from build123d import *

# Parameters (mm, degrees)
SKETCH_1_W          = 25
SKETCH_1_H          = 15
EXTRUDE_2_DEPTH     = 2
SKETCH_3_W          = 2
SKETCH_3_H          = 25
EXTRUDE_3_DEPTH     = 33
SKETCH_4_W          = 25
SKETCH_4_H          = 2
EXTRUDE_4_DEPTH     = 33
SKETCH_5_R          = 1
CUT_EXTRUDE_2_DEPTH = 71.75485849
SKETCH_6_R          = 1
CUT_EXTRUDE_3_DEPTH = 71.75485849
SKETCH_7_R          = 3
CUT_EXTRUDE_4_DEPTH = 71.75485849
SKETCH_8_R          = 3
CUT_EXTRUDE_5_DEPTH = 71.75485849
SKETCH_9_R          = 12.5
SKETCH_9_R_2        = 3
EXTRUDE_5_DEPTH     = 2
SKETCH_10_R         = 12.5
SKETCH_10_R_2       = 3
EXTRUDE_6_DEPTH     = 2
SKETCH_11_R         = 1
CUT_EXTRUDE_6_DEPTH = 71.75485849
SKETCH_12_R         = 12.5
SKETCH_12_R_2       = 3
EXTRUDE_7_DEPTH     = 2
EXTRUDE_START       = -2
SKETCH_13_R         = 12.5
SKETCH_13_R_2       = 3
EXTRUDE_8_DEPTH     = 2
SKETCH_14_R         = 1
CUT_EXTRUDE_7_DEPTH = 71.75485849


with BuildPart() as part:
    # 草图1 → 凸台-拉伸2 (new body)
    with BuildSketch(Plane.XY):
        Polygon((-12.5, 12.5), (-27.5, 12.5), (-27.5, -12.5), (-12.5, -12.5), (12.5, -12.5), (27.5, -12.5), (27.5, 12.5), (12.5, 12.5), align=None)
        with Locations((0, 20)):
            Rectangle(SKETCH_1_W, SKETCH_1_H)
        with Locations((0, -20)):
            Rectangle(SKETCH_1_W, SKETCH_1_H)
    extrude(amount=EXTRUDE_2_DEPTH)

    # 草图3 → 凸台-拉伸3 (add)
    with BuildSketch(Plane.XY.offset(2)):
        with Locations((26.5, 0)):
            Rectangle(SKETCH_3_W, SKETCH_3_H)
        with Locations((-26.5, 0)):
            Rectangle(SKETCH_3_W, SKETCH_3_H)
    extrude(amount=EXTRUDE_3_DEPTH)

    # 草图4 → 凸台-拉伸4 (add)
    with BuildSketch(Plane(origin=(0, 0, 0), x_dir=(-1, 0, 0), z_dir=(0, 0, -1))):
        with Locations((0, 26.5)):
            Rectangle(SKETCH_4_W, SKETCH_4_H)
        with Locations((0, -26.5)):
            Rectangle(SKETCH_4_W, SKETCH_4_H)
    extrude(amount=EXTRUDE_4_DEPTH)

    # 草图5 → 切除-拉伸2 (cut, through all)
    with BuildSketch(Plane.ZY.offset(27.5)):
        with BuildLine():
            Line((35, 12.5), (22.5, 12.5))
            ThreePointArc((22.5, 12.5), (31.338834765, 8.838834765), (35, 0))
            Line((35, 0), (35, 12.5))
        make_face()
        with BuildLine():
            Line((35, -12.5), (35, 0))
            ThreePointArc((35, 0), (31.338834765, -8.838834765), (22.5, -12.5))
            Line((22.5, -12.5), (35, -12.5))
        make_face()
        with Locations((29.682514636, 0)):
            Circle(SKETCH_5_R)
        with Locations((22.5, 6.957836122)):
            Circle(SKETCH_5_R)
        with Locations((15.317485364, 0)):
            Circle(SKETCH_5_R)
        with Locations((22.5, -6.957836122)):
            Circle(SKETCH_5_R)
    extrude(amount=-CUT_EXTRUDE_2_DEPTH, mode=Mode.SUBTRACT)

    # 草图6 → 切除-拉伸3 (cut, through all)
    with BuildSketch(Plane(origin=(0, 27.5, 0), x_dir=(1, 0, 0), z_dir=(0, 1, 0))):
        with BuildLine():
            Line((-12.5, 33), (-12.5, 20.5))
            ThreePointArc((-12.5, 20.5), (-8.838834765, 29.338834765), (0, 33))
            Line((0, 33), (-12.5, 33))
        make_face()
        with BuildLine():
            ThreePointArc((0, 33), (8.838834765, 29.338834765), (12.5, 20.5))
            Line((12.5, 20.5), (12.5, 33))
            Line((12.5, 33), (0, 33))
        make_face()
        with Locations(Location((6.473248516, 20.5, 0), (0, 0, 270))):
            Circle(SKETCH_6_R)
        with Locations(Location((0, 28.122142327, 0), (0, 0, 270))):
            Circle(SKETCH_6_R)
        with Locations(Location((-6.473248516, 20.5, 0), (0, 0, 270))):
            Circle(SKETCH_6_R)
        with Locations(Location((0, 12.877857673, 0), (0, 0, 270))):
            Circle(SKETCH_6_R)
    extrude(amount=-CUT_EXTRUDE_3_DEPTH, mode=Mode.SUBTRACT)

    # 草图7 → 切除-拉伸4 (cut, through all)
    with BuildSketch(Plane(origin=(0, 27.5, 0), x_dir=(1, 0, 0), z_dir=(0, 1, 0))):
        with Locations(Location((0, 20.5, 0), (0, 0, 270))):
            Circle(SKETCH_7_R)
    extrude(amount=-CUT_EXTRUDE_4_DEPTH, mode=Mode.SUBTRACT)

    # 草图8 → 切除-拉伸5 (cut, through all)
    with BuildSketch(Plane(origin=(27.5, 0, 0), x_dir=(0, 0, -1), z_dir=(1, 0, 0))):
        with Locations((-22.5, 0)):
            Circle(SKETCH_8_R)
    extrude(amount=-CUT_EXTRUDE_5_DEPTH, mode=Mode.SUBTRACT)

    # 草图9 → 凸台-拉伸5 (add)
    with BuildSketch(Plane(origin=(27.5, 0, 0), x_dir=(0, 0, -1), z_dir=(1, 0, 0))):
        with Locations((-22.5, 0)):
            Circle(SKETCH_9_R)
        with Locations((-22.5, 0)):
            Circle(SKETCH_9_R_2, mode=Mode.SUBTRACT)
    extrude(amount=-EXTRUDE_5_DEPTH)

    # 草图10 → 凸台-拉伸6 (add)
    with BuildSketch(Plane.ZY.offset(27.5)):
        with Locations((22.5, 0)):
            Circle(SKETCH_10_R)
        with Locations(Location((22.5, 0, 0), (0, 0, 180))):
            Circle(SKETCH_10_R_2, mode=Mode.SUBTRACT)
    extrude(amount=-EXTRUDE_6_DEPTH)

    # 草图11 → 切除-拉伸6 (cut, through all)
    with BuildSketch(Plane.ZY.offset(27.5)):
        with Locations((22.5, 7.071067812)):
            Circle(SKETCH_11_R)
        with Locations((29.571067812, 0)):
            Circle(SKETCH_11_R)
        with Locations(Location((22.5, -7.071067812, 0), (0, 0, 90))):
            Circle(SKETCH_11_R)
        with Locations(Location((15.428932188, 0, 0), (0, 0, 90))):
            Circle(SKETCH_11_R)
    extrude(amount=-CUT_EXTRUDE_6_DEPTH, mode=Mode.SUBTRACT)

    # 草图12 → 凸台-拉伸7 (add)
    with BuildSketch(Plane(origin=(0, 27.5, 0), x_dir=(1, 0, 0), z_dir=(0, 1, 0))):
        with Locations((0, 20.5)):
            Circle(SKETCH_12_R)
        with Locations(Location((0, 20.5, 0), (0, 0, 270))):
            Circle(SKETCH_12_R_2, mode=Mode.SUBTRACT)
    extrude(amount=-EXTRUDE_7_DEPTH)

    # 草图13 → 凸台-拉伸8 (add)
    with BuildSketch(Plane.XZ.offset(27.5).offset(EXTRUDE_START)):
        with Locations((0, -20.5)):
            Circle(SKETCH_13_R)
        with Locations(Location((0, -20.5, 0), (0, 0, 90))):
            Circle(SKETCH_13_R_2, mode=Mode.SUBTRACT)
    extrude(amount=EXTRUDE_8_DEPTH)

    # 草图14 → 切除-拉伸7 (cut, through all)
    with BuildSketch(Plane(origin=(0, -27.5, 0), x_dir=(-1, 0, 0), z_dir=(0, -1, 0))):
        with Locations(Location((0, 13.428932188, 0), (0, 0, 90))):
            Circle(SKETCH_14_R)
        with Locations(Location((-7.071067812, 20.5, 0), (0, 0, 90))):
            Circle(SKETCH_14_R)
        with Locations(Location((0, 27.571067812, 0), (0, 0, 90))):
            Circle(SKETCH_14_R)
        with Locations(Location((7.071067812, 20.5, 0), (0, 0, 90))):
            Circle(SKETCH_14_R)
    extrude(amount=-CUT_EXTRUDE_7_DEPTH, mode=Mode.SUBTRACT)


solid = part.part
Design review of the part built by this model. Coordinates are the model's own, in mm. A direction names the side the tool comes from. Coordinates: 2 decimals unless noted, no trailing zeros. Loops run counter-clockwise (first coordinate to the right, second up) from the corner with the lowest first, then second, coordinate; pieces in that order, holes last. Notation, with made-up numbers: (59, -7.5) - (74, -7.5) arc R23 ccw to (74, 24.5) - close; hole circle Ø8 at (77, -22). An arc over 180 degrees is marked (long way). Use CSV: the item, a comma, the result in double quotes. Start each with the question number.
1. Add section C-C on x = 17. Give the boundary of the cut face in (y, z), plus the area to 3 significant figures.
2. Add section A-A on z = -5.5. Give the boundary of the cut face in (x, y), plus the area to 3 significant figures.
3. To check wall thickness, follow probe 1 along Y at (x, z) = (27.1, 22.5); probe 2 along X at (y, z) = (-9.5, 24.5); probe 3 along Y at (x, z) = (-26, 22). State the ranges of each line that lie inside material, in increasing order.
4. For faces 1 (the flat face through (0, 0, 2)), 2 (the flat face through (-26, 12.5, 8)), 3 (the flat face through (26, 12.5, 8)), list the 3-axis set-ups (+Z, -Z, +X, -X, +Y, -Y) from which the entire face can be reached by the end or side of a thin tool; tool diameter is ignored.
5. Add section B-B on y = -4.5. Give the boundary of the cut face in (x, z).
6. Mouldability with a two-part tool opening along Y and no side actions: class faces 4 (the flat face through (-26, -12.5, 9)), 5 (the cylindrical face through (-26.5, 0.1, 25.5)), 6 (the flat face through (-12.5, 26, -6)) as released by +Y, released by -Y, zero draft, split by the parting line, or undercut.
7. Clearance check with flat-ended pins moving along their axes: pin 1 (4 mm diameter, centred on x = 7.5, y = 16, fed in from -Z); pin 2 (10 mm diameter, centred on x = -7.5, z = 4.5, fed in from -Y); pin 3 (8 mm diameter, centred on x = -4, y = 19, fed in from +Z). State where each tip first meets the part, or that it passes through.
Resolved:
1,outline,"(-12.5, 0) - (12.5, 0) - (12.5, 2) - (-12.5, 2) - close"
1,area,"50.0 mm2"
2,outline,"(-12.5, -27.5) - (12.5, -27.5) - (12.5, -25.5) - (-12.5, -25.5) - close; (-12.5, 25.5) - (12.5, 25.5) - (12.5, 27.5) - (-12.5, 27.5) - close"
2,area,"100 mm2"
3,probe 1,"-12.5 to -8.07, -6.07 to -3, 3 to 6.07, 8.07 to 12.5"
3,probe 2,"-27.5 to -25.5, 25.5 to 27.5"
3,probe 3,"-12.5 to -7.94, -6.21 to -2.96, 2.96 to 6.21, 7.94 to 12.5"
4,face 1,"+Z, +Y, -Y"
4,face 2,"+Z, -Z, -X, +Y"
4,face 3,"+Z, -Z, +X, +Y"
5,outline,"(-27.5, 0) - (27.5, 0) - (27.5, 34.16) - (25.5, 34.16) - (25.5, 2) - (-25.5, 2) - (-25.5, 34.16) - (-27.5, 34.16) - close"
6,face 4,"released by -Y"
6,face 5,"undercut"
6,face 6,"zero draft"
7,pin 1,"z = 0"
7,pin 2,"y = -27.5"
7,pin 3,"z = 2"
